from build123d import *

# Parameters (mm, degrees)
F0_W     = 133.35
F0_H     = 254
F1_DEPTH = 12.7
F3_DEPTH = 294
F5_DEPTH = 12.701


# Not quite as in the source:
# - an extrude ends at something that could not be found from the text; its depth is read off the source's solid
# - a pattern or mirror of a feature is missing from the dataset's text; its kind, count and spacing are read off the source's solid


with BuildPart() as f1:
    # F0 (on Front) → F1 (new body)
    with BuildSketch(Plane.XZ):
        Rectangle(F0_W, F0_H)
    extrude(amount=F1_DEPTH)

    # F0 (on Front) + F2 (on face) → F3 (cut, through all)
    with BuildSketch(Plane.XZ):
        Rectangle(F0_W, F0_H)
    with BuildSketch(Plane.XZ.offset(12.7)):
        with BuildLine():
            Line((-66.675, 73.025), (0, 73.025))
            ThreePointArc((0, 73.025), (9.525, 82.55), (0, 92.075))
            Line((0, 92.075), (-66.675, 92.075))
            Line((-66.675, 92.075), (-66.675, 73.025))
        make_face()
    extrude(amount=-F3_DEPTH, mode=Mode.SUBTRACT)

    # F4 (on face) → F5 (cut, through all)
    with BuildSketch(Plane.XZ.offset(12.7)):
        with BuildLine():
            Line((66.675, 127), (38.1, 127))
            Line((38.1, 127), (38.1, 50.8))
            ThreePointArc((38.1, 50.8), (45.4193088889, 4.1102242857), (66.675, -38.1))
            Line((66.675, -38.1), (66.675, 127))
        make_face()
    f5 = extrude(amount=-F5_DEPTH, mode=Mode.SUBTRACT)

    # F5_copies: F5 across plane
    add(f5.mirror(Plane(origin=(0, 0, 0), x_dir=(0, 0, -1), z_dir=(-1, 0, 0))), mode=Mode.SUBTRACT)


solid = f1.part
The listing builds one solid part. Answer for the finished solid, in the listing's coordinates (mm). A direction names the side the tool comes from. Give positions to 0.01 mm unless a question says otherwise; leave off trailing zeros. Write each loop counter-clockwise with the first axis right and the second up, starting at its lowest first coordinate (ties: lowest second). Pieces come first, ordered by that corner, then holes.
Item 1: Find the intervals of material crossed by line 1 along Z through (x, y) = (-34, -11.25) (3 decimals); line 2 along Z through (x, y) = (3, -7.5); line 3 along X through (y, z) = (-6.75, 35.5), in increasing order.
Item 2: Section B-B, the plane x = 4.5 is taken. Write down the section's boundary in (y, z).
Item 3: Section A-A, the plane y = -5 is taken. Write down the section's boundary in (x, z) (3 decimals), plus the area to 3 significant figures.
Item 4: Determine the mould class of faces 4 (the cylindrical face through (-45.22, -6.44, 4.74)), 5 (the flat face through (-19, -6, 92.075)), 6 (the flat face through (-38.1, -6, 62)), 7 (the flat face through (-1, -6, -127)) for opening direction Z: released by +Z, released by -Z, zero draft, split by the parting line, or undercut.
Item 5: Section D-D, the plane x = -56 is taken. Write down the section's boundary in (y, z).
Item 6: Section C-C, the plane z = 82.55 is taken. Write down the section's boundary in (x, y) (3 decimals), plus the area to 3 significant figures.
Item 7: Which of the six approach directions +Z, -Z, +X, -X, +Y, -Y give full straight-line access (tool end or side, diameter ignored) to faces 1 (the flat face through (38.1, -6, 89)), 2 (the flat face through (-19, -6, 73.025)), 3 (the flat face through (-38.1, -6, 110))?
Item 8: Flat-ended cylindrical pins translate along their axes: P1, Ø1, axis at y = -8.5, z = 70.5, coming from the +X side; P2, Ø10, axis at x = -51, z = -2.5, coming from the -Y side; P3, Ø4, axis at y = -5.5, z = 106, coming from the -X side; P4, Ø1, axis at y = -5.5, z = -16.5, coming from the +X side. Find the tip coordinate at first contact, or state that the pin passes through.
Completed:
1. line 1: z = -127 to 73.025, 92.075 to 127
1. line 2: z = -127 to 73.51, 91.59 to 127
1. line 3: x = -38.87 to 38.87
2. outline: (-12.7, -127) - (0, -127) - (0, 74.16) - (-12.7, 74.16) - close; (-12.7, 90.94) - (0, 90.94) - (0, 127) - (-12.7, 127) - close
3. outline: (-66.675, -127) - (66.675, -127) - (66.675, -38.1) arc R152.576 cw to (38.1, 50.8) - (38.1, 127) - (-38.1, 127) - (-38.1, 92.075) - (0, 92.075) arc R9.525 cw to (0, 73.025) - (-38.1, 73.025) - (-38.1, 50.8) arc R152.576 cw to (-66.675, -38.1) - close
3. area: 25,200 mm2
4. face 4: released by +Z
4. face 5: undercut
4. face 6: zero draft
4. face 7: released by -Z
5. outline: (-12.7, -127) - (0, -127) - (0, -20.91) - (-12.7, -20.91) - close
6. outline: (9.525, -12.7) - (38.1, -12.7) - (38.1, 0) - (9.525, 0) - close
6. area: 363 mm2
7. face 1: +Z, +X, +Y, -Y
7. face 2: -X, +Y, -Y
7. face 3: +Z, -X, +Y, -Y
8. P1: stops at x = 38.1
8. P2: stops at y = -12.7
8. P3: stops at x = -38.1
8. P4: stops at x = 53.99
